```python
from build123d import *

# Parameters (mm, degrees)
ESBO_O1_R                     = 30
RESSALTO_EXTRUS_O2_DEPTH      = 10
ESBO_O3_R                     = 12.494753049
RESSALTO_EXTRUS_O3_DEPTH      = 22
ESBO_O4_R                     = 30
ESBO_O4_R_2                   = 18.335840205
RESSALTO_EXTRUS_O4_DEPTH      = 51
ESBO_O5_R                     = 30
RESSALTO_EXTRUS_O5_DEPTH      = 10
ESBO_O6_R                     = 21.382326649
CORTE_EXTRUS_O1_DEPTH         = 2
ESBO_O7_R                     = 10.833594829
CORTE_EXTRUS_O2_DEPTH         = 2
ESBO_O8_W                     = 7.784469092
ESBO_O8_H                     = 33.042586886
CORTE_EXTRUS_O3_DEPTH         = 17
RESSALTO_EXTRUS_O7_DEPTH      = 17
ESBO_O11_W                    = 17.91144748
ESBO_O11_H                    = 4.730260337
CORTE_EXTRUS_O4_DEPTH         = 14
RESSALTO_EXTRUS_O9_DEPTH      = 29
RESSALTO_EXTRUS_O9_DEPTH_BACK = 24


with BuildPart() as part:
    # Esboço1 → Ressalto-extrusão2 (new body)
    with BuildSketch(Plane(origin=(0, 0, 0), x_dir=(1, 0, 0), z_dir=(0, 1, 0))):
        with Locations(Location((0, 0, 0), (0, 0, 270))):
            Circle(ESBO_O1_R)
    extrude(amount=RESSALTO_EXTRUS_O2_DEPTH)

    # Esboço3 → Ressalto-extrusão3 (add)
    with BuildSketch(Plane.XZ):
        with Locations(Location((0, 0, 0), (0, 0, 270))):
            Circle(ESBO_O3_R)
    extrude(amount=RESSALTO_EXTRUS_O3_DEPTH)

    # Esboço4 → Ressalto-extrusão4 (add)
    with BuildSketch(Plane(origin=(0, 10, 0), x_dir=(1, 0, 0), z_dir=(0, 1, 0))):
        with Locations(Location((0, 0, 0), (0, 0, 270))):
            Circle(ESBO_O4_R)
        with Locations(Location((0, 0, 0), (0, 0, 90))):
            Circle(ESBO_O4_R_2, mode=Mode.SUBTRACT)
    extrude(amount=RESSALTO_EXTRUS_O4_DEPTH)

    # Esboço5 → Ressalto-extrusão5 (add)
    with BuildSketch(Plane(origin=(0, 61, 0), x_dir=(1, 0, 0), z_dir=(0, 1, 0))):
        with Locations(Location((0, 0, 0), (0, 0, 270))):
            Circle(ESBO_O5_R)
    extrude(amount=RESSALTO_EXTRUS_O5_DEPTH)

    # Esboço6 → Corte-extrusão1 (cut)
    with BuildSketch(Plane(origin=(0, 71, 0), x_dir=(1, 0, 0), z_dir=(0, 1, 0))):
        with Locations(Location((0, 0, 0), (0, 0, 270))):
            Circle(ESBO_O6_R)
    extrude(amount=-CORTE_EXTRUS_O1_DEPTH, mode=Mode.SUBTRACT)

    # Esboço7 → Corte-extrusão2 (cut)
    with BuildSketch(Plane(origin=(0, 69, 0), x_dir=(1, 0, 0), z_dir=(0, 1, 0))):
        with Locations(Location((0, 0, 0), (0, 0, 270))):
            Circle(ESBO_O7_R)
    extrude(amount=-CORTE_EXTRUS_O2_DEPTH, mode=Mode.SUBTRACT)

    # Esboço8 → Corte-extrusão3 (cut)
    with BuildSketch(Plane.XZ.offset(22)):
        Rectangle(ESBO_O8_W, ESBO_O8_H)
    extrude(amount=-CORTE_EXTRUS_O3_DEPTH, mode=Mode.SUBTRACT)

    # Esboço10 → Ressalto-extrusão7 (add)
    with BuildSketch(Plane.XZ):
        with BuildLine():
            Line((-10, -30), (-10, -35.901739495))
            Line((-10, -35.901739495), (10, -35.901739495))
            Line((10, -35.901739495), (10, -30))
            Line((10, -30), (10, -28.284271247))
            ThreePointArc((10, -28.284271247), (0, -30), (-10, -28.284271247))
            Line((-10, -28.284271247), (-10, -30))
        make_face()
    extrude(amount=-RESSALTO_EXTRUS_O7_DEPTH)

    # Esboço11 → Corte-extrusão4 (cut)
    with BuildSketch(Plane.XZ):
        with Locations((-0.221595313, -32.668697771)):
            Rectangle(ESBO_O11_W, ESBO_O11_H)
    extrude(amount=-CORTE_EXTRUS_O4_DEPTH, mode=Mode.SUBTRACT)

    # Esboço13 → Ressalto-extrusão9 (add, two sides: drawn at the far end of the back side and taken through both)
    with BuildSketch(Plane(origin=(0, 30, 0), x_dir=(1, 0, 0), z_dir=(0, 1, 0)).offset(-RESSALTO_EXTRUS_O9_DEPTH_BACK)):
        with BuildLine():
            Line((-30, 22), (-43.507715599, 22))
            Line((-43.507715599, 22), (-43.507715599, -22))
            Line((-43.507715599, -22), (-30, -22))
            Line((-30, -22), (-20.396078054, -22))
            ThreePointArc((-20.396078054, -22), (30, 0), (-20.396078054, 22))
            Line((-20.396078054, 22), (-30, 22))
        make_face()
    extrude(amount=RESSALTO_EXTRUS_O9_DEPTH + RESSALTO_EXTRUS_O9_DEPTH_BACK)


solid = part.part
```
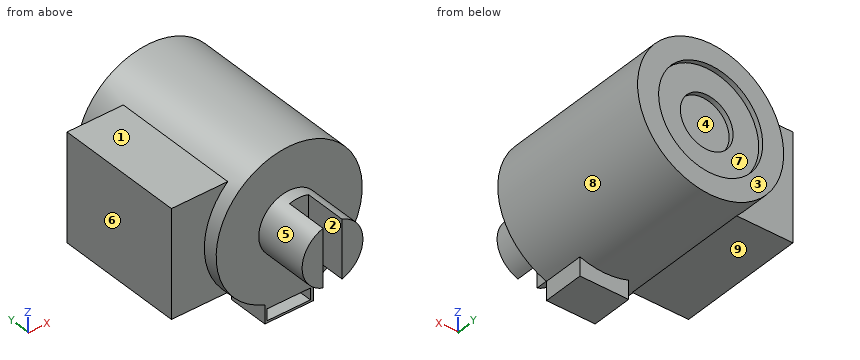
Geometry check sheet. Reference: the model listing, model coordinates, mm. Face numbers are marked on the shaded views. A direction names the side the tool comes from. Coordinates: 2 decimals unless noted, no trailing zeros. Order: outer loops, then holes, each group sorted by start corner. A loop starts at its lowest first (then second) coordinate and runs counter-clockwise, first axis right, second up.
Item 1: Section check D-D (z = 16). Enter the section's corners in (x, y).
Item 2: Section check C-C (y = 26). Enter the section's corners in (x, z), plus the area to 3 significant figures.
Item 3: Section check A-A (x = 0). Enter the section's corners in (y, z), plus the area to 3 significant figures.
Item 4: Tool access check on the marked faces 1, 2, 3, 4 and 5. Record the directions out of +Z, -Z, +X, -X, +Y, -Y that give a thin tool (end or side, any length) a straight path to the whole face; none if there is none.
Item 5: Section check B-B (z = 0). Enter the section's corners in (x, y).
Item 6: Scan lines: line 1 along X through (y, z) = (67.75, 0); line 2 along X through (y, z) = (59.9, 0); line 3 along Y through (x, z) = (-4.5, -11.5). Record each from-to range of solid material in increasing order.
Item 7: Mould release check, pull along X, two halves, no side actions. Record for the marked faces 6, 7, 8 and 9: released by +X, released by -X, zero draft, split by the parting line, or undercut.
Item 8: Depth check by flat-ended pin: pin 1 (4 mm diameter, centred on x = -2.5, z = 10, fed in from -Y); pin 2 (1.5 mm diameter, centred on x = 12, y = 36, fed in from +Z); pin 3 (1.4 mm diameter, centred on x = 3, z = -31.5, fed in from -Y); pin 4 (1.5 mm diameter, centred on x = -4.5, z = -23, fed in from -Y). Enter the tip coordinate at first touch or a pass-through.
Check sheet entries:
1. outline: (-43.51, 6) - (-25.38, 6) - (-25.38, 0) - (25.38, 0) - (25.38, 71) - (14.18, 71) - (14.18, 69) - (-14.18, 69) - (-14.18, 71) - (-25.38, 71) - (-25.38, 59) - (-43.51, 59) - close; hole (-8.96, 59) - (8.96, 59) - (8.96, 61) - (-8.96, 61) - close
2. outline: (-43.51, -22) - (-20.4, -22) arc R30 ccw (long way) to (-20.4, 22) - (-43.51, 22) - close
2. area: 3,550 mm2
3. outline: (-5, -12.49) - (0, -12.49) - (0, -30.3) - (14, -30.3) - (14, -35.03) - (0, -35.03) - (0, -35.9) - (17, -35.9) - (17, -30) - (71, -30) - (71, -21.38) - (69, -21.38) - (69, -10.83) - (67, -10.83) - (67, 10.83) - (69, 10.83) - (69, 21.38) - (71, 21.38) - (71, 30) - (0, 30) - (0, 12.49) - (-5, 12.49) - close; hole (59, -18.34) - (61, -18.34) - (61, 18.34) - (59, 18.34) - close
3. area: 4,220 mm2
4. face 1: +Z, -X, +Y, -Y
4. face 2: +Z, -Z, -Y
4. face 3: +Z, -Z, +X, -X, +Y
4. face 4: +Y
4. face 5: -Y
5. outline: (-43.51, 6) - (-30, 6) - (-30, 0) - (-12.49, 0) - (-12.49, -22) - (-3.89, -22) - (-3.89, -5) - (3.89, -5) - (3.89, -22) - (12.49, -22) - (12.49, 0) - (30, 0) - (30, 71) - (21.38, 71) - (21.38, 69) - (10.83, 69) - (10.83, 67) - (-10.83, 67) - (-10.83, 69) - (-21.38, 69) - (-21.38, 71) - (-30, 71) - (-30, 59) - (-43.51, 59) - close; hole (-18.34, 59) - (18.34, 59) - (18.34, 61) - (-18.34, 61) - close
6. line 1: x = -30 to -10.83, 10.83 to 30
6. line 2: x = -30 to -18.34, 18.34 to 30
6. line 3: y = -22 to 59, 61 to 69
7. face 6: released by -X
7. face 7: undercut
7. face 8: split by the parting line
7. face 9: zero draft
8. pin 1: stops at y = -22
8. pin 2: stops at z = 27.81
8. pin 3: stops at y = 14
8. pin 4: stops at y = 0
